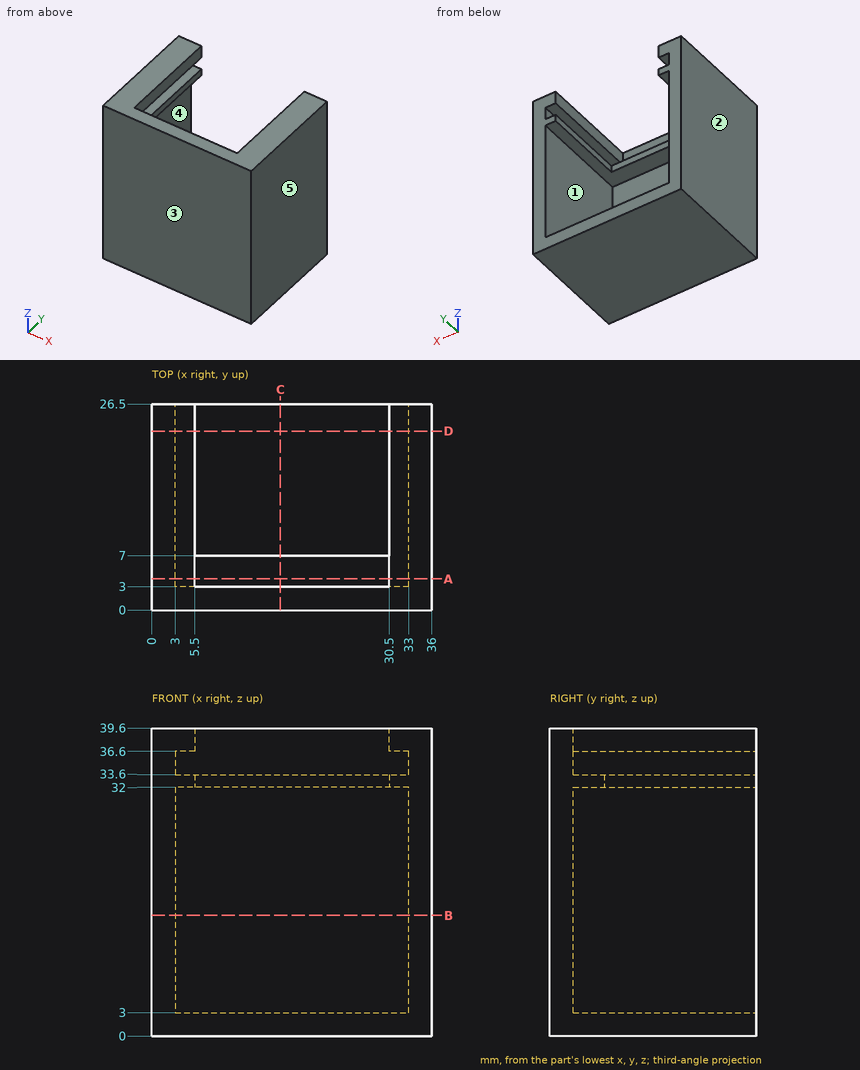
Here's the drawing with two shaded views (mm, measured from the low corner). I have some questions. A direction names the side the tool comes from. Give positions to 0.01 mm unless a question says otherwise; leave off trailing zeros. Order: outer loops, then holes, each group sorted by start corner. A loop starts at its lowest first (then second) coordinate and runs counter-clockwise, first axis right, second up. Notation, with made-up numbers: (-33.5, 61) - (0.5, 61) arc R23 ccw to (0.5, 83) - close; hole circle Ø8 at (-1.5, 0.5). An arc over 180 degrees is marked (long way). Use a Markdown table: item, result. Add a question column.
Q1. If we mould it in two halves opening along X, with no side actions, what happens to the marked faces 1, 2 and 3? For each: released by +X, released by -X, zero draft, split by the parting line, or undercut.
Q2. If we section it at B-B on z = 15.5: Write out the boundary of the cut face in (x, y).
Q3. Please list where these lines run through material, in increasing order: line 1 along X through (y, z) = (16.5, 14); line 2 along Z through (x, y) = (4.5, 7.25); line 3 along Z through (x, y) = (29.5, 3.75).
Q4. If we section it at A-A on y = 4: Write out the boundary of the cut face in (x, z).
Q5. On a 3-axis mill with a long thin cutter (end or side, diameter ignored), from which of +Z, -Z, +X, -X, +Y, -Y can I reach the whole of each face in a straight line? I mean the marked faces 4 and 5. Say none if no direction works.
Q6. If we section it at D-D on y = 23: Write out the boundary of the cut face in (x, z), plus the area to 3 significant figures.
Q7. If we section it at C-C on x = 16.5: Write out the boundary of the cut face in (y, z).
Q8. I'm going to push flat-ended pins straight in: pin 1 (3 mm diameter, centred on x = 18, z = 36, fed in from +Y); pin 2 (4 mm diameter, centred on x = 23, z = 35.5, fed in from +Y); pin 3 (7 mm diameter, centred on x = 24, y = 15.5, fed in from -Z); pin 4 (6 mm diameter, centred on x = 21, y = 16, fed in from +Z). Where does each tip first touch, or does it pass through?
Answers follow:
| question | item | result |
|---|---|---|
| 1 | face 1 | undercut |
| 1 | face 2 | released by -X |
| 1 | face 3 | zero draft |
| 2 | outline | (0, 0) - (36, 0) - (36, 26.5) - (33, 26.5) - (33, 3) - (3, 3) - (3, 26.5) - (0, 26.5) - close |
| 3 | line 1 | x = 0 to 3, 33 to 36 |
| 3 | line 2 | z = 0 to 3, 32 to 33.6, 36.6 to 39.6 |
| 3 | line 3 | z = 0 to 3, 32 to 33.6 |
| 4 | outline | (0, 0) - (36, 0) - (36, 39.6) - (30.5, 39.6) - (30.5, 36.6) - (33, 36.6) - (33, 33.6) - (3, 33.6) - (3, 36.6) - (5.5, 36.6) - (5.5, 39.6) - (0, 39.6) - close; hole (3, 3) - (33, 3) - (33, 32) - (3, 32) - close |
| 5 | face 4 | +Y |
| 5 | face 5 | +Z, -Z, +X, +Y, -Y |
| 6 | outline | (0, 0) - (36, 0) - (36, 39.6) - (30.5, 39.6) - (30.5, 36.6) - (33, 36.6) - (33, 33.6) - (30.5, 33.6) - (30.5, 32) - (33, 32) - (33, 3) - (3, 3) - (3, 32) - (5.5, 32) - (5.5, 33.6) - (3, 33.6) - (3, 36.6) - (5.5, 36.6) - (5.5, 39.6) - (0, 39.6) - close |
| 6 | area | 351 mm^2 |
| 7 | outline | (0, 0) - (26.5, 0) - (26.5, 3) - (3, 3) - (3, 32) - (7, 32) - (7, 33.6) - (3, 33.6) - (3, 39.6) - (0, 39.6) - close |
| 8 | pin 1 | stops at y = 3 |
| 8 | pin 2 | stops at y = 7 |
| 8 | pin 3 | stops at z = 0 |
| 8 | pin 4 | stops at z = 3 |
